```python
from build123d import *

# Parameters (mm, degrees)
SKETCH1_W           = 100
SKETCH1_H           = 20
BOSS_EXTRUDE1_DEPTH = 40
SKETCH2_R           = 4
CUT_EXTRUDE1_DEPTH  = 110.544511501
SKETCH3_R           = 8
CUT_EXTRUDE2_DEPTH  = 110.544511501
CUT_EXTRUDE3_DEPTH  = 109.480412979
CHAMFER1_SIZE       = 5


with BuildPart() as part:
    # Sketch1 → Boss-Extrude1 (new body)
    with BuildSketch(Plane(origin=(0, 0, 0), x_dir=(1, 0, 0), z_dir=(0, 1, 0))):
        with Locations((50, 10)):
            Rectangle(SKETCH1_W, SKETCH1_H)
    extrude(amount=BOSS_EXTRUDE1_DEPTH)

    # Sketch2 → Cut-Extrude1 (cut, through all)
    with BuildSketch(Plane(origin=(0, 40, 0), x_dir=(1, 0, 0), z_dir=(0, 1, 0))):
        with Locations(Location((10, 10, 0), (0, 0, 270))):
            Circle(SKETCH2_R)
        with Locations(Location((90, 10, 0), (0, 0, 270))):
            Circle(SKETCH2_R)
    extrude(amount=-CUT_EXTRUDE1_DEPTH, mode=Mode.SUBTRACT)

    # Sketch3 → Cut-Extrude2 (cut, through all)
    with BuildSketch(Plane(origin=(0, 0, -20), x_dir=(-1, 0, 0), z_dir=(0, 0, -1))):
        with Locations((-50, 20)):
            Circle(SKETCH3_R)
    extrude(amount=-CUT_EXTRUDE2_DEPTH, mode=Mode.SUBTRACT)

    # 3DSketch1 → Cut-Extrude3 (cut, through all)
    with BuildSketch(Plane(origin=(100, 38, -18), x_dir=(0, -0.913811548620257, 0.4061384660534479), z_dir=(-1, 0, 0))):
        Polygon((0, 0), (6.498215457, 14.620984778), (39.395431207, 0), (32.89721575, -14.620984778), align=None)
    extrude(amount=CUT_EXTRUDE3_DEPTH, mode=Mode.SUBTRACT)

    # Chamfer1
    # the kernel refuses this chamfer: 5 mm, written as the material it takes off along each edge
    with BuildSketch(Plane(origin=(100, -12.85841494, -20), x_dir=(0.0274958766105877, 0, 0.9996219169112968), z_dir=(0, 1, 0)), Plane(origin=(100, -12.85841494, 0), x_dir=(-0.9996219169112968, 0, 0.027495876610586334), z_dir=(0, 1, 0))) as chamfer1_piece_1:
        Polygon((CHAMFER1_SIZE * 0.999621916911, -CHAMFER1_SIZE * 0.0274958766106), (-CHAMFER1_SIZE * 0.0274958766106, -CHAMFER1_SIZE * 0.999621916911), (0, 0), align=None)
    extrude(amount=65.71682988, mode=Mode.SUBTRACT)
    with BuildSketch(Plane(origin=(0, -12.85841494, -20), x_dir=(-0.027495876610586372, 0, 0.9996219169112968), z_dir=(0, 1, 0)), Plane(origin=(0, -12.85841494, 0), x_dir=(0.9996219169112968, 0, 0.027495876610586372), z_dir=(0, 1, 0))) as chamfer1_piece_2:
        Polygon((CHAMFER1_SIZE * 0.999621916911, CHAMFER1_SIZE * 0.0274958766106), (-CHAMFER1_SIZE * 0.0274958766106, CHAMFER1_SIZE * 0.999621916911), (0, 0), align=None)
    extrude(amount=65.71682988, mode=Mode.SUBTRACT)


solid = part.part
```
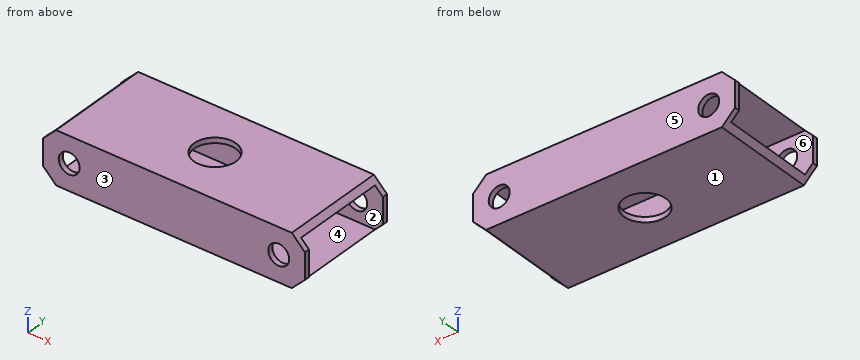
Part model, mm, in its own coordinate system. Face numbers are marked on the shaded views. A direction names the side the tool comes from. Round coordinates to 2 decimals unless told otherwise and drop trailing zeros. Loops run counter-clockwise (first coordinate to the right, second up) from the corner with the lowest first, then second, coordinate; pieces in that order, holes last.
Item 1: Drill centre lines: line 1 (X direction, y = 1.1, z = -10); line 2 (Y direction, x = 50, z = -1.45); line 3 (Y direction, x = 49, z = -10.5). Where is each one in solid material? Low to high.
Item 2: 3-axis set-ups, long thin cutter, end or side, ignore diameter. For the marked faces 5 and 6: which of +Z, -Z, +X, -X, +Y, -Y reach the whole face in a straight line?
Item 3: Cut at A-A, the plane y = 20. Give the cut face in (x, z).
Item 4: Cut at C-C, the plane z = -16.25. Give the cut face in (x, y), then the cut area to 3 significant figures.
Item 5: Cut at B-B, the plane x = 50. Give the cut face in (y, z), then the cut area to 3 significant figures.
Item 6: Cut at D-D, the plane y = 31.5. Give the cut face in (x, z), then the cut area to 3 significant figures.
Item 7: Mould opens along Y. For the marked faces 1, 2, 3 and 4 say: +Y half, -Y half, draft (parallel to the pull), parting line (faces both ways), or undercut.
Item 8: Drop flat-ended pins along their axis: P1, Ø1, axis at y = 25, z = -2, coming from the -X side; P2, Ø5, axis at x = 65, z = -10, coming from the -Y side. Give the stop position or say it passes through.
A:
1. line 1: x = 0 to 6, 14 to 86, 94 to 100
1. line 2: y = 0 to 12, 28 to 40
1. line 3: y = 0 to 2, 38 to 40
2. face 5: +Z, -Z, +X, -X, +Y
2. face 6: +X, -X
3. outline: (3, -18) - (5, -20) - (42, -20) - (42, -18) - close; (3, -2) - (42, -2) - (42, 0) - (5, 0) - close; (58, -20) - (95, -20) - (97, -18) - (58, -18) - close; (58, -2) - (97, -2) - (95, 0) - (58, 0) - close
4. outline: (1.25, 0) - (98.75, 0) - (98.75, 2) - (1.25, 2) - close; (1.25, 38) - (98.75, 38) - (98.75, 40) - (1.25, 40) - close
4. area: 390 mm2
5. outline: (0, -20) - (12, -20) - (12, -18) - (2, -18) - (2, -2) - (12, -2) - (12, 0) - (0, 0) - close; (28, -20) - (40, -20) - (40, 0) - (28, 0) - (28, -2) - (38, -2) - (38, -18) - (28, -18) - close
5. area: 160 mm2
6. outline: (3, -18) - (5, -20) - (95, -20) - (97, -18) - close; (3, -2) - (97, -2) - (95, 0) - (5, 0) - close
6. area: 368 mm2
7. face 1: draft
7. face 2: undercut
7. face 3: -Y half
7. face 4: undercut
8. P1: stops at x = 3
8. P2: stops at y = 0
